Can you work these out from the drawing? Everything is in mm from the part's minimum corner. A direction names the side the tool comes from. Give positions to 0.01 mm unless a question says otherwise; leave off trailing zeros. Loops run counter-clockwise (first coordinate to the right, second up) from the corner with the lowest first, then second, coordinate; pieces in that order, holes last.
Q1. If we section it at A-A (y = 6.5): Please give me the cut outline in (x, z).
Q2. If we section it at D-D (y = 3): Please give me the cut outline in (x, z).
Q3. For the marked faces 4, 5 and 6, which set-ups out of +Z, -Z, +X, -X, +Y, -Y let a thin tool reach every point of the face, with its end or its side?
Q4. We'd pull the mould along Z, two halves only. Please class the marked faces 1, 2 and 3: +Z half, -Z half, draft (parallel to the pull), parting line (faces both ways), or undercut.
Q5. If we section it at B-B (z = 63.2): Please give me the cut outline in (x, y).
Q6. Will these pins go through, and if not, where does the flat tip stop? P1, Ø3.5, axis at x = 2.5, z = 6.5, coming from the +Y side; P2, Ø4, axis at x = 7.5, y = 4, coming from the -Z side; P3, Ø1.5, axis at x = 21, y = 3, coming from the +Z side; P4, Ø4, axis at y = 7, z = 61.5, coming from the -X side.
Q7. If we section it at C-C (x = 15.25): Please give me the cut outline in (y, z).
Q8. I need wall thicknesses on line 1 (X direction, y = 0.75, z = 6.5); line 2 (Z direction, x = 24.5, y = 0.4); line 3 (Z direction, x = 10, y = 10.75). Which ranges of each line are inside material? Lowest first, please.
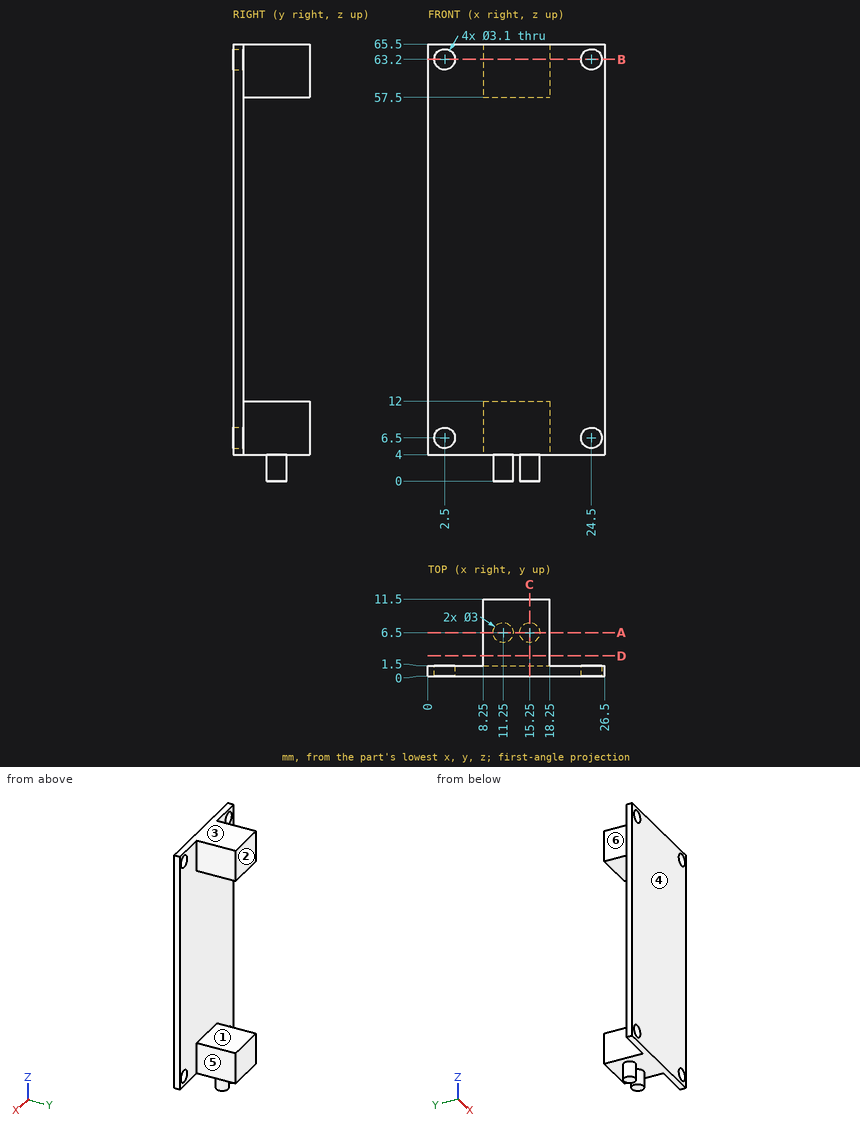
Check sheet entries:
1. outline: (8.25, 4) - (9.75, 4) - (9.75, 0) - (12.75, 0) - (12.75, 4) - (13.75, 4) - (13.75, 0) - (16.75, 0) - (16.75, 4) - (18.25, 4) - (18.25, 12) - (8.25, 12) - close; (8.25, 57.5) - (18.25, 57.5) - (18.25, 65.5) - (8.25, 65.5) - close
2. outline: (8.25, 4) - (18.25, 4) - (18.25, 12) - (8.25, 12) - close; (8.25, 57.5) - (18.25, 57.5) - (18.25, 65.5) - (8.25, 65.5) - close
3. face 4: +Z, -Z, +X, -X, -Y
3. face 5: +Z, -Z, +X, +Y
3. face 6: +Z, -Z, -X, +Y
4. face 1: undercut
4. face 2: draft
4. face 3: +Z half
5. outline: (0, 0) - (0.95, 0) - (0.95, 1.5) - (0, 1.5) - close; (4.05, 0) - (22.95, 0) - (22.95, 1.5) - (18.25, 1.5) - (18.25, 11.5) - (8.25, 11.5) - (8.25, 1.5) - (4.05, 1.5) - close; (26.05, 0) - (26.5, 0) - (26.5, 1.5) - (26.05, 1.5) - close
6. P1: stops at y = 1.5
6. P2: stops at z = 4
6. P3: passes through
6. P4: stops at x = 8.25
7. outline: (0, 4) - (5, 4) - (5, 0) - (8, 0) - (8, 4) - (11.5, 4) - (11.5, 12) - (1.5, 12) - (1.5, 57.5) - (11.5, 57.5) - (11.5, 65.5) - (0, 65.5) - close
8. line 1: x = 0 to 0.95, 4.05 to 22.95, 26.05 to 26.5
8. line 2: z = 4 to 4.95, 8.05 to 61.65, 64.75 to 65.5
8. line 3: z = 4 to 12, 57.5 to 65.5
